Autodesk Inventor part; units mm, degrees
ref_plane "Work Plane1" through (6.35, 0, 0) normal (1, 0, 0) x (0, 1, 0)
ref_plane "XZ Plane" through (0, 0, 0) normal (0, 1, 0) x (-1, 0, 0)
ref_plane "XY Plane" through (0, 0, 0) normal (0, 0, 1) x (1, 0, 0)
sketch "Sketch1" plane through (0, 0, 0) normal (0, 0, 1) x (1, 0, 0)
  circle A0 centre (0, 0) radius 3.175
  circle A1 centre (0, 0) radius 5.08
  dimension "d0" = 6.35
  dimension "d1" = 10.16
extrude "Extrusion1" add sketch "Sketch1" along normal blind 12.7
chamfer "Chamfer1" distance 0.508 angle 45 2 edges at (-5.08, 0, 12.7) (-5.08, 0, 0)
ref_plane "Work Plane1" through (6.35, 0, 0) normal (1, 0, 0) x (0, 1, 0)
sketch "Sketch2" plane through (6.35, 0, 0) normal (1, 0, 0) x (0, 1, 0)
  circle A0 centre (0, 6.35) radius 1.1282
  point P0 (0, 0)
  dimension "d8" = 6.35
hole "Hole1" at (6.35, 0, 6.35) direction (-1, 0, 0) diameter 2.1565 depth 6.35
properties part number "Carriage Axle Set Screw Holder"
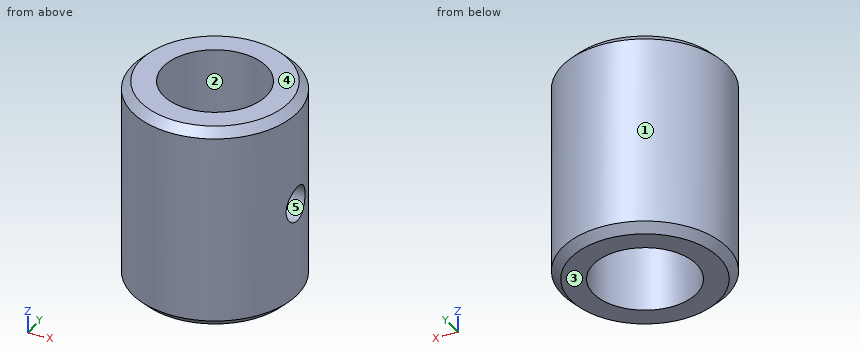
Part model, mm, in its own coordinate system. Face numbers are marked on the shaded views. A direction names the side the tool comes from. Give positions to 0.01 mm unless a question says otherwise; leave off trailing zeros. Write each loop counter-clockwise with the first axis right and the second up, starting at its lowest first coordinate (ties: lowest second). Pieces come first, ordered by that corner, then holes.
1) Probe L1, parallel to Y at x = 0, z = 6.25 (3 decimals); L2, parallel to X at y = 2.5, z = 5.5; L3, parallel to Y at x = -1.5, z = 3.5. List the from-to ranges inside material, lowest first.
Resolved:
L1: y = -5.08 to -3.175, 3.175 to 5.08
L2: x = -4.42 to -1.96, 1.96 to 4.42
L3: y = -4.85 to -2.8, 2.8 to 4.85
2) Cut at A-A on x = 0. Write the cut outline in (y, z) (3 decimals).
Resolved:
outline: (-5.08, 0.508) - (-4.572, 0) - (-3.175, 0) - (-3.175, 12.7) - (-4.572, 12.7) - (-5.08, 12.192) - close; (3.175, 0) - (4.572, 0) - (5.08, 0.508) - (5.08, 12.192) - (4.572, 12.7) - (3.175, 12.7) - close
3) Pin check, flat tip, straight feed: pin 1 (1 mm diameter, centred on x = -2, z = 11.5, fed in from +Y). Stop position of the tip, or through.
Resolved:
pin 1: stops at y = 4.85
4) Which spindle directions (+Z, -Z, +X, -X, +Y, -Y) get a long thin tool onto all of the face, cutting with end or side? Do the marked faces 4 and 5. Say none if no direction does.
Resolved:
face 4: +Z, +X, -X, +Y, -Y
face 5: +X
5) Cut at D-D on z = 5.75. Write the cut outline in (x, y) (3 decimals).
Resolved:
outline: (3.046, -0.896) arc R3.175 cw (long way) to (3.046, 0.896) - (5, 0.896) arc R5.08 ccw (long way) to (5, -0.896) - close
6) Cut at C-C on z = 2.75. Write the cut outline in (x, y) (3 decimals), then the cut area to 3 significant figures.
Resolved:
outline: circle Ø10.16 at (0, 0); hole circle Ø6.35 at (0, 0)
area: 49.4 mm2
7) Cut at B-B on y = 0. Write the cut outline in (x, z) (3 decimals), then the cut area to 3 significant figures.
Resolved:
outline: (-5.08, 0.508) - (-4.572, 0) - (-3.175, 0) - (-3.175, 12.7) - (-4.572, 12.7) - (-5.08, 12.192) - close; (3.175, 0) - (4.572, 0) - (5.08, 0.508) - (5.08, 5.272) - (3.175, 5.272) - close; (3.175, 7.428) - (5.08, 7.428) - (5.08, 12.192) - (4.572, 12.7) - (3.175, 12.7) - close
area: 43.8 mm2
8) Two-plate mould, pull along Y, no slides. Class the marked faces 1, 2 and 3: released by +Y, released by -Y, zero draft, split by the parting line, or undercut.
Resolved:
face 1: split by the parting line
face 2: undercut
face 3: zero draft
